Autodesk Inventor part; units mm, degrees
ref_plane "YZ Plane" through (0, 0, 0) normal (1, 0, 0) x (0, 1, 0)
ref_plane "XZ Plane" through (0, 0, 0) normal (0, 1, 0) x (-1, 0, 0)
ref_plane "XY Plane" through (0, 0, 0) normal (0, 0, 1) x (1, 0, 0)
sketch "Sketch1" plane through (0, 0, 0) normal (0, 0, 1) x (1, 0, 0)
  circle A0 centre (0, 0) radius 80
  circle A1 centre (0, 0) radius 55
  line L0 (-7.5, 73) -> (7.5, 73)
  line L1 (7.5, 73) -> (7.5, 70)
  line L2 (7.5, 70) -> (-7.5, 70)
  line L3 (-7.5, 70) -> (-7.5, 73)
  line L4 (-66.9699, 30.0048) -> (-59.4699, 42.9952)
  line L5 (-59.4699, 42.9952) -> (-56.8718, 41.4952)
  line L6 (-56.8718, 41.4952) -> (-64.3718, 28.5048)
  line L7 (-64.3718, 28.5048) -> (-66.9699, 30.0048)
  line L8 (-59.4699, -42.9952) -> (-66.9699, -30.0048)
  line L9 (-66.9699, -30.0048) -> (-64.3718, -28.5048)
  line L10 (-64.3718, -28.5048) -> (-56.8718, -41.4952)
  line L11 (-56.8718, -41.4952) -> (-59.4699, -42.9952)
  line L12 (7.5, -73) -> (-7.5, -73)
  line L13 (-7.5, -73) -> (-7.5, -70)
  line L14 (-7.5, -70) -> (7.5, -70)
  line L15 (7.5, -70) -> (7.5, -73)
  line L16 (66.9699, -30.0048) -> (59.4699, -42.9952)
  line L17 (59.4699, -42.9952) -> (56.8718, -41.4952)
  line L18 (56.8718, -41.4952) -> (64.3718, -28.5048)
  line L19 (64.3718, -28.5048) -> (66.9699, -30.0048)
  line L20 (59.4699, 42.9952) -> (66.9699, 30.0048)
  line L21 (66.9699, 30.0048) -> (64.3718, 28.5048)
  line L22 (64.3718, 28.5048) -> (56.8718, 41.4952)
  line L23 (56.8718, 41.4952) -> (59.4699, 42.9952)
  line L24 (-58.1708, 43.7452) -> (-43.1708, 43.7452)
  line L25 (-43.1708, 43.7452) -> (-43.1708, 40.7452)
  line L26 (-43.1708, 40.7452) -> (-58.1708, 40.7452)
  line L27 (-58.1708, 40.7452) -> (-58.1708, 43.7452)
  line L28 (-58.1708, -40.7452) -> (-43.1708, -40.7452)
  line L29 (-43.1708, -40.7452) -> (-43.1708, -43.7452)
  line L30 (-43.1708, -43.7452) -> (-58.1708, -43.7452)
  line L31 (-58.1708, -43.7452) -> (-58.1708, -40.7452)
  line L32 (0, 20) -> (-100, 20)
  line L33 (-100, 20) -> (-100, -20)
  line L34 (-100, -20) -> (0, -20)
  line L35 (0, -20) -> (0, 20)
  point P0 (0, 73)
  point P1 (7.5, 71.5)
  point P2 (0, 70)
  point P3 (-63.2199, 36.5)
  point P4 (-58.1708, 42.2452)
  point P5 (-60.6218, 35)
  point P6 (-63.2199, -36.5)
  point P7 (-65.6708, -29.2548)
  point P8 (-60.6218, -35)
  point P9 (0, -73)
  point P10 (-7.5, -71.5)
  point P11 (0, -70)
  point P12 (63.2199, -36.5)
  point P13 (58.1708, -42.2452)
  point P14 (60.6218, -35)
  point P15 (63.2199, 36.5)
  point P16 (65.6708, 29.2548)
  point P17 (60.6218, 35)
  point P18 (-58.1708, 42.2452)
  point P19 (-58.1708, -42.2452)
  point P20 (-51.2348, -20)
  point P21 (-77.4597, -20)
  point P22 (-77.4597, 20)
  point P23 (-51.2348, 20)
  dimension "d0" = 160
  dimension "d1" = 110
  dimension "d2" = 15
  dimension "d3" = 3
  dimension "d11" = 70
  dimension "d14" = 360
  dimension "d18" = 15
  dimension "d19" = 3
  dimension "d20" = 15
  dimension "d21" = 3
  dimension "d22" = 40
  dimension "d23" = 100
extrude "Extrusion2" add sketch "Sketch1" along normal blind 6 contours A0 L34 A1 L32 | L27 L24 L25 L26 L6 L5 | L11 L10 L28 L29 L30 L31 picked at (16.7927, -65.9701)
sketch "草圖2" plane through (0, 0, 6) normal (0, 0, 1) x (1, 0, 0)
  arc A0 (-51.2348, -20) -> (-51.2348, 20) centre (0, 0) ccw
  circle A1 centre (0, 0) radius 55
  circle A2 centre (0, 0) radius 57
  circle A3 centre (0, 0) radius 60
  circle A4 centre (0, 0) radius 62
  arc A5 (-77.4597, -20) -> (-77.4597, 20) centre (0, 0) ccw
  line L0 (-51.2348, 20) -> (-77.4597, 20)
  line L1 (-51.2348, -20) -> (-77.4597, -20)
  line L2 (-51.2348, -20) -> (-77.4597, -20)
  line L3 (-51.2348, 20) -> (-77.4597, 20)
  line L4 (-77.4597, 20) -> (-77.4597, 22)
  line L5 (-77.4597, 22) -> (-51.2348, 22)
  line L6 (-51.2348, 22) -> (-51.2348, 20)
  line L7 (-77.4597, -20) -> (-51.2348, -20)
  line L8 (-51.2348, -20) -> (-51.2348, -22)
  line L9 (-51.2348, -22) -> (-77.4597, -22)
  line L10 (-77.4597, -22) -> (-77.4597, -20)
  point P0 (-58.6856, 20)
  point P1 (-58.6856, -20)
  point P2 (-55.8211, 22)
  point P3 (-55.8211, -22)
  point P4 (-52.5833, -22)
  point P5 (-52.5833, 22)
  point P6 (-57.9655, -22)
  point P7 (-76.9155, -22)
  point P8 (-76.9155, 22)
  point P9 (-57.9655, 22)
  dimension "d24" = 114
  dimension "d25" = 120
  dimension "d26" = 124
  dimension "d27" = 2
  dimension "d28" = 26.2249
  dimension "d29" = 2
  dimension "d30" = 26.2249
extrude "擠出3" add sketch "草圖2" against normal blind 8.5 contours L8 L9 A2 L1 | A0 L6 L5 A2 L9 L8 | L0 A2 L5 L6 | A2 L9 A3 L1 | L0 A3 L5 A2 | A3 L9 A4 L1 | L0 A4 L5 A3 | A3 L5 A4 L9
extrude "擠出4" add sketch "草圖2" along normal blind 2.5 contours L8 L9 A2 L1 | A0 L6 L5 A2 L9 L8 | L0 A2 L5 L6 | A2 L9 A3 L1 | L0 A3 L5 A2 | A3 L9 A4 L1 | L0 A4 L5 A3 | A3 L5 A4 L9 | A4 L9 A5 L1 | L0 A5 L5 A4 | A4 L5 A5 L9
sketch "草圖3" plane through (0, 0, 0) normal (0, 0, -1) x (-1, 0, 0)
  line L0 (-63, 3) -> (-66, 3)
  line L1 (-66, 3) -> (-66, -3)
  line L2 (-66, -3) -> (-63, -3)
  line L3 (-63, -3) -> (-63, 3)
  line L4 (-34.0981, -53.0596) -> (-35.5981, -55.6577)
  line L5 (-35.5981, -55.6577) -> (-30.4019, -58.6577)
  line L6 (-30.4019, -58.6577) -> (-28.9019, -56.0596)
  line L7 (-28.9019, -56.0596) -> (-34.0981, -53.0596)
  line L8 (28.9019, -56.0596) -> (30.4019, -58.6577)
  line L9 (30.4019, -58.6577) -> (35.5981, -55.6577)
  line L10 (35.5981, -55.6577) -> (34.0981, -53.0596)
  line L11 (34.0981, -53.0596) -> (28.9019, -56.0596)
  line L12 (63, -3) -> (66, -3)
  line L13 (66, -3) -> (66, 3)
  line L14 (66, 3) -> (63, 3)
  line L15 (63, 3) -> (63, -3)
  line L16 (34.0981, 53.0596) -> (35.5981, 55.6577)
  line L17 (35.5981, 55.6577) -> (30.4019, 58.6577)
  line L18 (30.4019, 58.6577) -> (28.9019, 56.0596)
  line L19 (28.9019, 56.0596) -> (34.0981, 53.0596)
  line L20 (-28.9019, 56.0596) -> (-30.4019, 58.6577)
  line L21 (-30.4019, 58.6577) -> (-35.5981, 55.6577)
  line L22 (-35.5981, 55.6577) -> (-34.0981, 53.0596)
  line L23 (-34.0981, 53.0596) -> (-28.9019, 56.0596)
  point P0 (0, 0)
  point P1 (-63, 0)
  point P2 (-31.5, -54.5596)
  point P3 (31.5, -54.5596)
  point P4 (63, 0)
  point P5 (31.5, 54.5596)
  point P6 (-31.5, 54.5596)
  dimension "d35" = 3
  dimension "d36" = 6
  dimension "d38" = 63
  dimension "d39" = 3
  dimension "d44" = 360
extrude "擠出5" cut sketch "草圖3" against normal through all contours L3 L2 L1 L0 | L7 L6 L5 L4 | L11 L10 L9 L8 | L19 L18 L17 L16 | L23 L22 L21 L20
extrude "擠出6" cut sketch "Sketch1" along normal through all contours L0 L1 L2 L3 | L4 L5 L27 L26 L6 L7 | L5 L6 L26 L27 | L8 L9 L10 L28 L31 L11 | L31 L28 L10 L11 | L12 L13 L14 L15 | L16 L17 L18 L19 | L20 L21 L22 L23
properties part number "back_cir_hold"
Work out the finished part from the listing and answer in its coordinate system (mm). A direction names the side the tool comes from. Round coordinates to 2 decimals unless told otherwise and drop trailing zeros. One line per item, written item: value.
Q1. Straight lines are drawn through the part: line 1 (Y direction, x = 0, z = 3.7); line 2 (Y direction, x = 0, z = 7); line 3 (Y direction, x = -65, z = 1.5). For each, find the intervals that lie inside material, in ascending order.
Derived:
line 1: -80 to -73, -70 to -55, 55 to 70, 73 to 80
line 2: -80 to -73, -70 to -60, -57 to -55, 55 to 57, 60 to 70, 73 to 80
line 3: -46.64 to -33.42, -28.87 to -20, 20 to 28.87, 33.42 to 46.64
Q2. Flat-ended cylindrical pins translate along their axes: pin 1 (1.5 mm diameter, centred on y = 2, z = 3.5, fed in from +X); pin 2 (5.5 mm diameter, centred on x = -61, z = 0.5, fed in from -Y); pin 3 (6 mm diameter, centred on y = 59, z = 5, fed in from +X). Find the tip coordinate at first contact, or state that the pin passes through.
Derived:
pin 1: x = 79.99
pin 2: y = -54.84
pin 3: x = 57.13
Q3. Determine the mould class of faces 1 (the face through (0, -73, 4)), 2 (the face through (48, -41, 0)), 3 (the face through (79.935, 3.235, 7.232)) for opening direction Y: released by +Y, released by -Y, zero draft, split by the parting line, or undercut.
Derived:
face 1: undercut
face 2: zero draft
face 3: split by the parting line
Q4. Find section B-B on z = 3.5. Give the number of separate pieces and of enclosed holes in the cut face, then the cut area to 3 significant figures.
Derived:
separate pieces: 1
enclosed holes: 11
area: 9,230 mm²
Q5. For faces 4 (the face through (58, 0, 0)), 5 (the face through (-60.57, 35.09, 4.19)), determine the directions among +Z, -Z, +X, -X, +Y, -Y from which every point of the face is accessible in a straight line to the end or side of a thin tool.
Derived:
face 4: -Z
face 5: +Z, -Z
